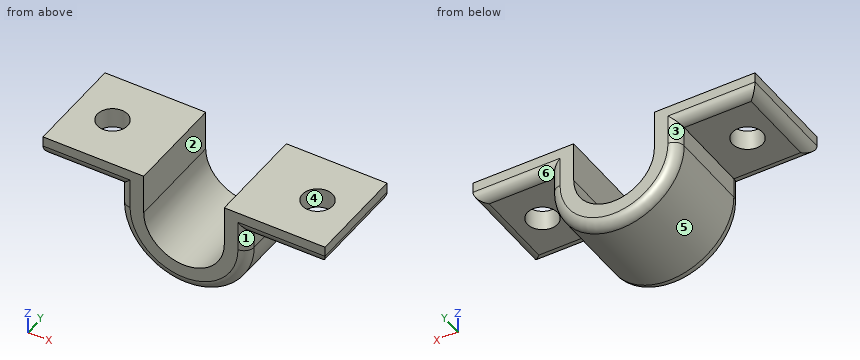
Autodesk Inventor part; units mm, degrees
ref_plane "YZ Plane" through (0, 0, 0) normal (1, 0, 0) x (0, 1, 0)
ref_plane "XZ Plane" through (0, 0, 0) normal (0, 1, 0) x (-1, 0, 0)
ref_plane "XY Plane" through (0, 0, 0) normal (0, 0, 1) x (1, 0, 0)
sketch "Sketch1" plane through (0, 0, 0) normal (0, 1, 0) x (-1, 0, 0)
  arc A0 (-4, 0) -> (4, 0) centre (0, 0) ccw
  line L0 (-4, 4) -> (-14, 4)
  line L1 (4, 4) -> (14, 4)
  line L2 (14, 2) -> (6.3562, 2)
  line L3 (-6.3562, 2) -> (-14, 2)
  line L4 (4, 0) -> (4, 4)
  line L5 (-4, 0) -> (-4, 4)
  line L6 (6.3562, 0) -> (6.3562, 2)
  line L7 (-6.3562, 0) -> (-6.3562, 2)
  arc A1 (-6.3562, 0) -> (6.3562, 0) centre (0, 0) ccw
  line L8 (14, 2) -> (14, 4)
  line L9 (-14, 2) -> (-14, 4)
  dimension "d0" = 8
  dimension "d2" = 2
  dimension "d3" = 10
  dimension "d4" = 10
  dimension "d5" = 6.3562
  dimension "d6" = 2
extrude "Extrusion1" add sketch "Sketch1" along normal mid plane 10
sketch "Sketch2" plane through (14, 5, 2) normal (0, 0, -1) x (-1, 0, 0)
  line L0 (0, -10) -> (0, 0)
  line L1 (0, 0) -> (7.6438, 0)
  point P0 (14, -5)
  point P1 (3.8219, -5)
  point P2 (0, -5)
  point P3 (3.8219, 0)
hole "Hole1" at (10.1781, 0, 2) direction (0, 0, 1) diameter 3 depth 2
mirror "Mirror1" about plane through (0, 0, 0) normal (1, 0, 0) of "Hole1"
fillet "Fillet1" radius 1 12 edges at (10.1781, 5, 2) (14, 0, 2) (10.1781, -5, 2) (-10.1781, 5, 2) (-14, 0, 2) (-10.1781, -5, 2) (-6.3562, 5, 1) (6.3562, 5, 1) (0, 5, -6.3562) (6.3562, -5, 1) (-6.3562, -5, 1) (0, -5, -6.3562)
properties part number "Part_B5"
Here's how the part is built. I have some questions about the finished solid (model axes, mm). Face numbers are marked on the shaded views. A direction names the side the tool comes from. Round coordinates to 2 decimals unless told otherwise and drop trailing zeros. Write each loop counter-clockwise with the first axis right and the second up, starting at its lowest first coordinate (ties: lowest second). Pieces come first, ordered by that corner, then holes.
Q1. Which directions (+Z, -Z, +X, -X, +Y, -Y) give clear straight access to the entire face, cutting with the end or side of a thin tool? Please do the marked faces 1, 2 and 3.
Q2. If we section it at B-B on x = -7.25: Write out the boundary of the cut face in (y, z).
Q3. Will these pins go through, and if not, where does the flat tip stop? P1, Ø1, axis at x = 2.5, y = -2, coming from the +Z side; P2, Ø3, axis at y = 1, z = -1.5, coming from the -X side; P3, Ø3.5, axis at x = 10, y = -1.5, coming from the -Z side; P4, Ø1.8, axis at x = 10.18, y = 0, coming from the +Z side.
Q4. If we section it at C-C on x = 0: Write out the boundary of the cut face in (y, z).
Q5. If we section it at A-A on y = 0: Write out the boundary of the cut face in (x, z), plus the area to 3 significant figures.
Q6. Please list where these lines run through material, in increasing order: probe 1 along X at (y, z) = (0, 2.9); probe 2 along X at (y, z) = (-2.75, 3); probe 3 along X at (y, z) = (0, 2.65).
Q7. If we mould it in two halves opening along Y, with no side actions, what happens to the marked faces 4, 5 and 6? For each: +Y half, -Y half, draft (parallel to the pull), parting line (faces both ways), or undercut.
Answer below:
1. face 1: -Z, +X, -Y
1. face 2: +Z, +Y, -Y
1. face 3: -Z, -X, +Y
2. outline: (-5, 3) arc R1 ccw to (-4, 2) - (4, 2) arc R1 ccw to (5, 3) - (5, 4) - (-5, 4) - close
3. P1: stops at z = -2.65
3. P2: stops at x = -6.36
3. P3: stops at z = 2
3. P4: passes through
4. outline: (-5, -5.36) arc R1 ccw to (-4, -6.36) - (4, -6.36) arc R1 ccw to (5, -5.36) - (5, -4) - (-5, -4) - close
5. outline: (-14, 3) arc R1 ccw to (-13, 2) - (-11.68, 2) - (-11.68, 4) - (-14, 4) - close; (-8.68, 2) - (-6.36, 2) - (-6.36, 0) arc R6.36 ccw to (6.36, 0) - (6.36, 2) - (8.68, 2) - (8.68, 4) - (4, 4) - (4, 0) arc R4 cw to (-4, 0) - (-4, 4) - (-8.68, 4) - close; (11.68, 2) - (13, 2) arc R1 ccw to (14, 3) - (14, 4) - (11.68, 4) - close
5. area: 75.3 mm2
6. probe 1: x = -13.99 to -11.68, -8.68 to -4, 4 to 8.68, 11.68 to 13.99
6. probe 2: x = -14 to -4, 4 to 14
6. probe 3: x = -13.94 to -11.68, -8.68 to -4, 4 to 8.68, 11.68 to 13.94
7. face 4: undercut
7. face 5: draft
7. face 6: +Y half
